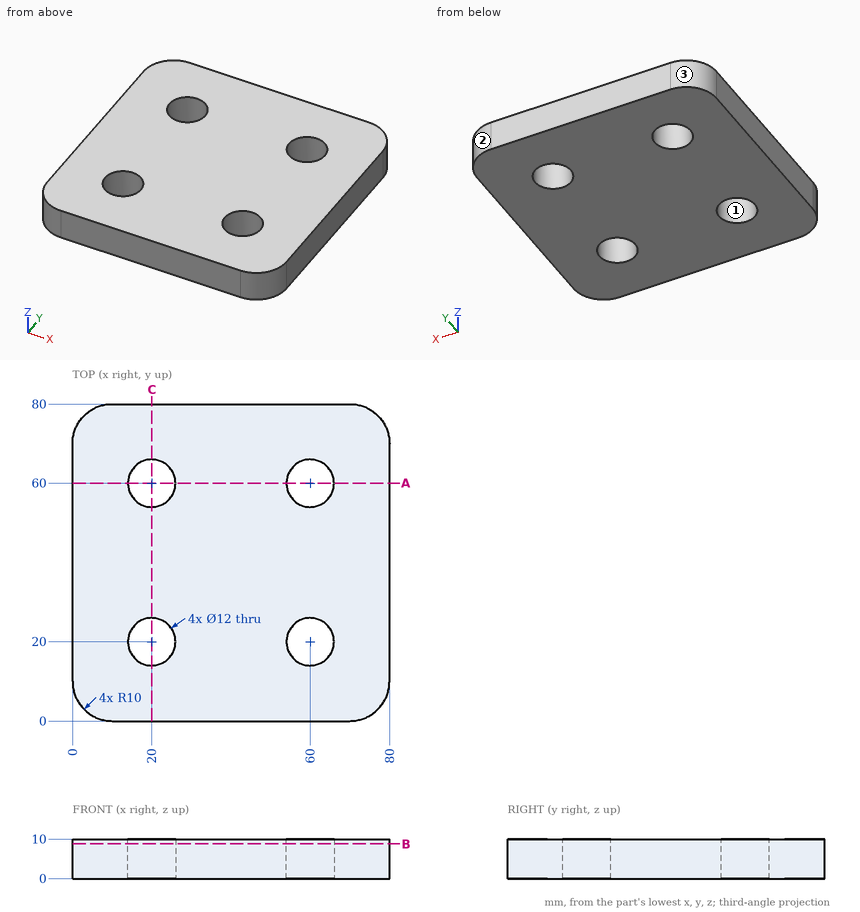
Here's the drawing with two shaded views (mm, measured from the low corner). I have some questions. Round coordinates to 2 decimals unless told otherwise and drop trailing zeros. Loops run counter-clockwise (first coordinate to the right, second up) from the corner with the lowest first, then second, coordinate; pieces in that order, holes last. Notation, with made-up numbers: (-10.5, 22.5) - (41.5, 22.5) arc R28 ccw to (41.5, 42.5) - close; hole circle Ø8 at (6.5, 47). An arc over 180 degrees is marked (long way). Write item = value, one per line.
1) If we mould it in two halves opening along X, with no side actions, what happens to the marked faces 1, 2 and 3? For each: pulls with the +X half, pulls with the -X half, needs draft (parallel to the pull), parting line crosses it, or undercut.
Computed:
face_1 = undercut
face_2 = pulls with the +X half
face_3 = pulls with the -X half
2) Imagine slicing it at A-A (y = 60). Please give me the cut outline in (x, z).
Computed:
outline = (0, 0) - (14, 0) - (14, 10) - (0, 10) - close; (26, 0) - (54, 0) - (54, 10) - (26, 10) - close; (66, 0) - (80, 0) - (80, 10) - (66, 10) - close
3) I need wall thicknesses on line 1 along Y through (x, z) = (20, 5.75); line 2 along X through (y, z) = (24, 8.5); line 3 along X through (y, z) = (58, 7.75). Which ranges of each line are inside material? Lowest first, please. Write a range as from..to.
Computed:
line_1 = 0..14, 26..54, 66..80
line_2 = 0..15.53, 24.47..55.53, 64.47..80
line_3 = 0..14.34, 25.66..54.34, 65.66..80
4) Imagine slicing it at B-B (z = 8.75). Please give me the cut outline in (x, y).
Computed:
outline = (0, 10) arc R10 ccw to (10, 0) - (70, 0) arc R10 ccw to (80, 10) - (80, 70) arc R10 ccw to (70, 80) - (10, 80) arc R10 ccw to (0, 70) - close; hole circle Ø12 at (20, 20); hole circle Ø12 at (20, 60); hole circle Ø12 at (60, 20); hole circle Ø12 at (60, 60)
